CAD build for the part. Positions are in the model's coordinates, mm. Coordinates: 2 decimals unless noted, no trailing zeros. Write each loop counter-clockwise with the first axis right and the second up, starting at its lowest first coordinate (ties: lowest second). Pieces come first, ordered by that corner, then holes. Notation, with made-up numbers: (-1.5, -38.75) - (3.5, -38.75) arc R19 ccw to (3.5, -4.75) - close; hole circle Ø4 at (88.25, -5.75). An arc over 180 degrees is marked (long way). One line per question, with ' | ' between items. Start each with the question number.
1. Probe line 1 (X direction, y = 2.5, z = 0.5); line 2 (Z direction, x = 30, y = 8.75); line 3 (Z direction, x = 32.5, y = 9). List the from-to ranges inside material, lowest first.
2. Band-saw the part on B-B, the plane x = 32.5. Write the cut outline in (y, z).
3. Two-plate mould, pull along Z, no slides. Class faces 1 (the cylindrical face through (-65.958, 5.916, -39.837)), 2 (the flat face through (-1, 12, -1)), 3 (the flat face through (-37.265, 10.521, 63.332)): +Z half, -Z half, draft (parallel to the pull), parting line (faces both ways), or undercut.
4. Band-saw the part on A-A, the plane z = 0. Write the cut outline in (x, y), then the cut area to 3 significant figures.
5. Band-saw the part on C-C, the plane x = 65. Write the cut outline in (y, z), then the cut area to 3 significant figures.
6. Band-saw the part on D-D, the plane y = 4.75. Give the number of separate pieces and of enclosed holes in the cut face, then the cut area to 3 significant figures.
7. Flat gauge pins, fed straight in: P1, Ø3, axis at x = -65, z = -37.53, coming from the +Y side; P2, Ø6, axis at x = 59, y = 10, coming from the -Z side; P3, Ø1, axis at x = -8, y = 5.5, coming from the -Z side; P4, Ø2, axis at x = 5, y = 7, coming from the -Z side. Where does each tip first touch, or does it go through?
from build123d import *

# Parameters (mm, degrees)
EXTRUDE_1_DEPTH     = 12
CHAMFER_1_SIZE      = 3
SKETCH_2_R          = 4
CUT_EXTRUDE_1_DEPTH = 13
M6X1_0_1_D          = 5


with BuildPart() as part:
    # 草圖1 → 填料-伸長1 (new body)
    with BuildSketch(Plane(origin=(0, 0, 0), x_dir=(1, 0, 0), z_dir=(0, 1, 0))):
        Polygon((0, 86.602540378), (-75, 43.301270189), (-75, -43.301270189), (0, -86.602540378), (75, -43.301270189), (75, 43.301270189), align=None)
    extrude(amount=EXTRUDE_1_DEPTH)

    # 導角1
    chamfer_1_edges = [part.edges().sort_by_distance(p)[0] for p in [
        (-75, 12, 0),
        (-37.5, 12, 64.951905284),
        (37.5, 12, 64.951905284),
        (75, 12, 0),
        (37.5, 12, -64.951905284),
        (-37.5, 12, -64.951905284),
    ]]
    chamfer(chamfer_1_edges, length=CHAMFER_1_SIZE)

    # 草圖2 → 除料-伸長1 (cut, through all)
    with BuildSketch(Plane(origin=(0, 12, 0), x_dir=(1, 0, 0), z_dir=(0, 1, 0))):
        with Locations((32.5, 56.291651246)):
            Circle(SKETCH_2_R)
        with Locations((32.5, -56.291651246)):
            Circle(SKETCH_2_R)
        with Locations((65, 0)):
            Circle(SKETCH_2_R)
        with Locations((-65, 0)):
            Circle(SKETCH_2_R)
        with Locations((-32.5, 56.291651246)):
            Circle(SKETCH_2_R)
        with Locations((-32.5, -56.291651246)):
            Circle(SKETCH_2_R)
    extrude(amount=-CUT_EXTRUDE_1_DEPTH, mode=Mode.SUBTRACT)

    # M6x1.0 螺紋孔1 (through all)
    with Locations(Plane(origin=(-65, 12, -37.527767497), x_dir=(0, 0, 1), z_dir=(0, 1, 0))):
        with Locations((0, 0), (-37.527767498, 65), (0, 130), (75.055534994, 130), (112.583302492, 65), (75.055534994, 0)):
            Hole(M6X1_0_1_D / 2)


solid = part.part
Filled in:
1) line 1: x = -75 to -68.97, -61.03 to 61.03, 68.97 to 75 | line 2: z = -69.28 to -59.41, -53.17 to 53.17, 59.41 to 69.28 | line 3: z = -67.84 to -60.29, -52.29 to 52.29, 60.29 to 67.84
2) outline: (0, -67.84) - (9, -67.84) - (12, -64.37) - (12, -60.29) - (0, -60.29) - close; (0, -52.29) - (12, -52.29) - (12, 52.29) - (0, 52.29) - close; (0, 60.29) - (12, 60.29) - (12, 64.37) - (9, 67.84) - (0, 67.84) - close
3) face 1: undercut | face 2: draft | face 3: +Z half
4) outline: (-75, 0) - (-69, 0) - (-69, 12) - (-72, 12) - (-75, 9) - close; (-61, 0) - (61, 0) - (61, 12) - (-61, 12) - close; (69, 0) - (75, 0) - (75, 9) - (72, 12) - (69, 12) - close | area: 1,600 mm²
5) outline: (0, -49.07) - (9, -49.07) - (12, -45.61) - (12, -40.03) - (0, -40.03) - close; (0, -35.03) - (12, -35.03) - (12, -4) - (0, -4) - close; (0, 4) - (12, 4) - (12, 35.03) - (0, 35.03) - close; (0, 40.03) - (12, 40.03) - (12, 45.61) - (9, 49.07) - (0, 49.07) - close | area: 951 mm²
6) separate pieces: 1 | enclosed holes: 12 | area: 19,100 mm²
7) P1: passes through | P2: stops at z = -54.17 | P3: stops at z = -82.27 | P4: stops at z = -84.29
